The model under review builds one solid part; all positions refer to its coordinate system, in mm. Coordinates: 2 decimals unless noted, no trailing zeros. Order: outer loops, then holes, each group sorted by start corner. A loop starts at its lowest first (then second) coordinate and runs counter-clockwise, first axis right, second up. Notation, with made-up numbers: M 65,52.25 L 88,52.25 A35 cw 88,87.25 Z; hole C 8,7 d11. An arc over 180 degrees is marked long. Answer in a Markdown table with one row per item.
Autodesk Inventor part; units mm, degrees
ref_plane "YZ Plane" through (0, 0, 0) normal (1, 0, 0) x (0, 1, 0)
ref_plane "XZ Plane" through (0, 0, 0) normal (0, 1, 0) x (-1, 0, 0)
ref_plane "XY Plane" through (0, 0, 0) normal (0, 0, 1) x (1, 0, 0)
sketch "Sketch1" plane through (0, 0, 0) normal (0, 1, 0) x (-1, 0, 0)
  line L0 (4.3325, 36.172) -> (109.3325, 36.172)
  line L1 (134.3325, 36.172) -> (247.3325, 36.172)
  line L2 (277.3325, 36.172) -> (277.3325, 33.172)
  line L3 (277.3325, 33.172) -> (280.3325, 33.172)
  line L4 (280.3325, 33.172) -> (280.3325, 19.172)
  line L5 (280.3325, 19.172) -> (277.3325, 19.172)
  line L6 (277.3325, 19.172) -> (277.3325, 16.172)
  line L7 (201.8325, -13.828) -> (201.8325, -16.828)
  line L8 (201.8325, -16.828) -> (226.8325, -16.828)
  line L9 (226.8325, -16.828) -> (226.8325, -13.828)
  line L10 (56.8325, -13.828) -> (56.8325, -16.828)
  line L11 (56.8325, -16.828) -> (81.8325, -16.828)
  line L12 (81.8325, -16.828) -> (81.8325, -13.828)
  line L13 (81.8325, -13.828) -> (201.8325, -13.828)
  line L14 (56.8325, -13.828) -> (46.8325, -13.828)
  line L15 (46.8325, -13.828) -> (46.8325, 11.172)
  arc A0 (46.8325, 11.172) -> (41.8325, 16.172) centre (41.8325, 11.172) ccw
  line L16 (41.8325, 16.172) -> (4.3325, 16.172)
  arc A1 (2.3325, 18.172) -> (4.3325, 16.172) centre (4.3325, 18.172) ccw
  line L17 (2.3325, 18.172) -> (2.3325, 34.172)
  arc A2 (4.3325, 36.172) -> (2.3325, 34.172) centre (4.3325, 34.172) ccw
  line L18 (5.4325, 19.172) -> (8.2325, 19.172)
  line L19 (8.2325, 19.172) -> (8.2325, 33.172)
  line L20 (8.2325, 33.172) -> (5.4325, 33.172)
  line L21 (5.4325, 33.172) -> (5.4325, 19.172)
  line L22 (109.3325, 36.172) -> (109.3325, 39.172)
  line L23 (109.3325, 39.172) -> (134.3325, 39.172)
  line L24 (134.3325, 39.172) -> (134.3325, 36.172)
  line L25 (277.3325, 36.172) -> (272.3325, 36.172)
  line L26 (272.3325, 36.172) -> (272.3325, 39.172)
  line L27 (272.3325, 39.172) -> (247.3325, 39.172)
  line L28 (247.3325, 39.172) -> (247.3325, 36.172)
  line L29 (226.8325, -13.828) -> (228.3045, -13.828)
  line L30 (277.3325, 16.172) -> (275.8605, 16.172)
  arc A3 (275.8605, 16.172) -> (273.0655, 15.3179) centre (275.8605, 11.172) ccw
  line L31 (273.0655, 15.3179) -> (231.0995, -12.9739)
  arc A4 (228.3045, -13.828) -> (231.0995, -12.9739) centre (228.3045, -8.828) ccw
extrude "Extrusion1" add sketch "Sketch1" along normal blind 3
properties part number "sideWallRight" material "Polycarbonate, Clear"
(1) Take a section at A-A (x = -21). Write out the cut boundary in (y, z).
Report:
| item | result |
|---|---|
| outline | M 0,16.17 L 3,16.17 L 3,36.17 L 0,36.17 Z |
(2) Insertion check: P1, Ø0.9, axis at x = -16, y = 1.5, coming from the -Z side; P2, Ø0.9, axis at y = 2, z = 34.5, coming from the -X side; P3, Ø1.5, axis at x = -165, y = 2, coming from the +Z side. Each pin has a flat end and moves straight along its axis. Give the tip position at first contact, or say it passes through.
Report:
| item | result |
|---|---|
| P1 | z = 16.17 |
| P2 | x = -277.33 |
| P3 | z = 36.17 |
(3) To check wall thickness, follow line 1 (X direction, y = 2.5, z = 25.5); line 2 (Z direction, x = -135, y = 1.2); line 3 (Z direction, x = -23.5, y = 1.05). State the ranges of each line that lie inside material, in increasing order. Write a range as [from, to].
Report:
| item | result |
|---|---|
| line 1 | [-280.33, -8.23], [-5.43, -2.33] |
| line 2 | [-13.83, 36.17] |
| line 3 | [16.17, 36.17] |
(4) Take a section at B-B (z = -1). Write out the cut boundary in (x, y).
Report:
| item | result |
|---|---|
| outline | M -248.86,0 L -46.83,0 L -46.83,3 L -248.86,3 Z |
